The listing builds one solid part. Answer for the finished solid, in the listing's coordinates (mm). A direction names the side the tool comes from. Give positions to 0.01 mm unless a question says otherwise; leave off trailing zeros. Order: outer loops, then holes, each group sorted by start corner. A loop starts at its lowest first (then second) coordinate and runs counter-clockwise, first axis right, second up. Notation, with made-up numbers: (72, 29) -> (126, 29) arc R24 cw to (126, 60) -> close; hole circle Ø11 at (42.25, -21.5). An arc over 180 degrees is marked (long way). Write item = value, one per line. Start each with the question number.
```python
from build123d import *

# Parameters (mm, degrees)
SKETCH_R      = 4.15
PAD_DEPTH     = 3
SKETCH001_R   = 5.3
SKETCH001_R_2 = 4.15
PAD001_DEPTH  = 10


with BuildPart() as part:
    # Sketch → Pad (new body)
    with BuildSketch(Plane.XY):
        with BuildLine():
            Line((5.368659, -3), (27.964674, -3))
            ThreePointArc((27.964674, -3), (33.333333, -6.15), (38.701992, -3))
            Line((38.701992, -3), (61.298007, -3))
            ThreePointArc((61.298007, -3), (66.666666, -6.15), (72.035325, -3))
            Line((72.035325, -3), (94.63134, -3))
            ThreePointArc((94.63134, -3), (99.999999, -6.15), (105.368658, -3))
            Line((105.368658, -3), (127.964673, -3))
            ThreePointArc((127.964673, -3), (133.333332, -6.15), (138.701991, -3))
            Line((138.701991, -3), (161.298006, -3))
            ThreePointArc((161.298006, -3), (166.666665, -6.15), (172.035324, -3))
            Line((172.035324, -3), (194.631339, -3))
            ThreePointArc((194.631339, -3), (199.999998, -6.15), (205.368657, -3))
            Line((205.368657, -3), (227.964672, -3))
            ThreePointArc((227.964672, -3), (239.483331, 0), (227.964672, 3))
            Line((205.368657, 3), (227.964672, 3))
            ThreePointArc((205.368657, 3), (199.999998, 6.15), (194.631339, 3))
            Line((172.035324, 3), (194.631339, 3))
            ThreePointArc((172.035324, 3), (166.666665, 6.15), (161.298006, 3))
            Line((138.701991, 3), (161.298006, 3))
            ThreePointArc((138.701991, 3), (133.333332, 6.15), (127.964673, 3))
            Line((105.368658, 3), (127.964673, 3))
            ThreePointArc((105.368658, 3), (99.999999, 6.15), (94.63134, 3))
            Line((72.035325, 3), (94.63134, 3))
            ThreePointArc((72.035325, 3), (66.666666, 6.15), (61.298007, 3))
            Line((38.701992, 3), (61.298007, 3))
            ThreePointArc((38.701992, 3), (33.333333, 6.15), (27.964674, 3))
            Line((5.368659, 3), (27.964674, 3))
            ThreePointArc((5.368659, 3), (-6.15, 0), (5.368659, -3))
        make_face()
        Circle(SKETCH_R, mode=Mode.SUBTRACT)
        with Locations((33.333333, 0)):
            Circle(SKETCH_R, mode=Mode.SUBTRACT)
        with Locations((66.666666, 0)):
            Circle(SKETCH_R, mode=Mode.SUBTRACT)
        with Locations((99.999999, 0)):
            Circle(SKETCH_R, mode=Mode.SUBTRACT)
        with Locations((133.333332, 0)):
            Circle(SKETCH_R, mode=Mode.SUBTRACT)
        with Locations((166.666665, 0)):
            Circle(SKETCH_R, mode=Mode.SUBTRACT)
        with Locations((199.999998, 0)):
            Circle(SKETCH_R, mode=Mode.SUBTRACT)
        with Locations((233.333331, 0)):
            Circle(SKETCH_R, mode=Mode.SUBTRACT)
    extrude(amount=PAD_DEPTH)

    # Sketch001 (on Face38 of Pad) → Pad001 (join)
    with BuildSketch(Plane.XY.offset(3)):
        Circle(SKETCH001_R)
        Circle(SKETCH001_R_2, mode=Mode.SUBTRACT)
        with Locations((33.333333, 0)):
            Circle(SKETCH001_R)
        with Locations((33.333333, 0)):
            Circle(SKETCH001_R_2, mode=Mode.SUBTRACT)
        with Locations((66.666666, 0)):
            Circle(SKETCH001_R)
        with Locations((66.666666, 0)):
            Circle(SKETCH001_R_2, mode=Mode.SUBTRACT)
        with Locations((99.999999, 0)):
            Circle(SKETCH001_R)
        with Locations((99.999999, 0)):
            Circle(SKETCH001_R_2, mode=Mode.SUBTRACT)
        with Locations((133.333332, 0)):
            Circle(SKETCH001_R)
        with Locations((133.333332, 0)):
            Circle(SKETCH001_R_2, mode=Mode.SUBTRACT)
        with Locations((166.666665, 0)):
            Circle(SKETCH001_R)
        with Locations((166.666665, 0)):
            Circle(SKETCH001_R_2, mode=Mode.SUBTRACT)
        with Locations((199.999998, 0)):
            Circle(SKETCH001_R)
        with Locations((199.999998, 0)):
            Circle(SKETCH001_R_2, mode=Mode.SUBTRACT)
        with Locations((233.333331, 0)):
            Circle(SKETCH001_R)
        with Locations((233.333331, 0)):
            Circle(SKETCH001_R_2, mode=Mode.SUBTRACT)
    extrude(amount=PAD001_DEPTH)


solid = part.part
```
Item 1: A cutting plane is placed at B-B, the plane z = 11. Count the separate pieces of the cut face and the enclosed holes in it, plus the area to 3 significant figures.
Item 2: Consider L1, parallel to Y at x = 100, z = 5.5; L2, parallel to Y at x = 40.5, z = 1.5; L3, parallel to Z at x = 117.5, y = 1.75. Determine where each line is inside the solid, lowest interval first. Write a range as from..to.
Item 3: Which of the six approach directions +Z, -Z, +X, -X, +Y, -Y give full straight-line access (tool end or side, diameter ignored) to faces 1 (the cylindrical face through (161.37, 0.23, 7.93)), 2 (the cylindrical face through (237.29, 1.25, 6.41))?
Item 4: Flat-ended cylindrical pins translate along their axes: pin 1 (2.5 mm diameter, centred on x = 46.5, z = 1.5, fed in from +Y); pin 2 (1 mm diameter, centred on y = -2.5, z = 6.5, fed in from -X); pin 3 (5 mm diameter, centred on y = 2.5, z = 6.5, fed in from -X); pin 4 (6.5 mm diameter, centred on x = 200, y = 0, fed in from +Z). Find the tip coordinate at first contact, or state that the pin passes through.
Item 5: A cutting plane is placed at A-A, the plane x = 100. Write down the section's boundary in (y, z), plus the area to 3 significant figures.
Item 6: The mould has two halves that part along Y. Classify faces 3 (the cylindrical face through (162.52, 0.18, 6.41)), 4 (the cylindrical face through (4.896, -2.03, 7.93)), 5 (the flat face through (202, -4, 13)): +Y half, -Y half, draft (parallel to the pull), parting line (faces both ways), or undercut.
Check values:
q1.separate_pieces = 8
q1.enclosed_holes = 8
q1.area = 273 mm^2
q2.L1 = -5.3..-4.15, 4.15..5.3
q2.L2 = -3..3
q2.L3 = 0..3
q3.face_1 = +Z
q3.face_2 = +Z, -Z
q4.pin_1 = 3
q4.pin_2 = -4.91
q4.pin_3 = -5.3
q4.pin_4 = through
q5.outline = (-6.15, 0) -> (-4.15, 0) -> (-4.15, 13) -> (-5.3, 13) -> (-5.3, 3) -> (-6.15, 3) -> close; (4.15, 0) -> (6.15, 0) -> (6.15, 3) -> (5.3, 3) -> (5.3, 13) -> (4.15, 13) -> close
q5.area = 35.0 mm^2
q6.face_3 = undercut
q6.face_4 = parting line
q6.face_5 = draft
